Here's how the part is built. I have some questions about the finished solid (model axes, mm). A direction names the side the tool comes from. Coordinates: 2 decimals unless noted, no trailing zeros. Loops run counter-clockwise (first coordinate to the right, second up) from the corner with the lowest first, then second, coordinate; pieces in that order, holes last. Notation, with made-up numbers: (44, -27) - (70, -27) arc R24 ccw to (70, 7) - close; hole circle Ø6 at (43.5, 24). An arc over 180 degrees is marked (long way). Use a Markdown table: item, result.
```python
from build123d import *

# Parameters (mm, degrees)
F0_W     = 90
F0_H     = 90
F1_DEPTH = 3
F0_H_2   = 30
F2_DEPTH = 90
F3_DEPTH = 100
F4_DEPTH = 80


with BuildPart() as f1:
    # F0 (on Right) → F1 (new body)
    with BuildSketch(Plane.YZ):
        Polygon((264.885695, 154.677426), (34.885695, 154.677426), (34.885695, 0.538323), (199.884153, 0.538323), (199.884153, -1.461677), (163.329955, -1.461677), (163.329955, -31.461677), (73.329955, -31.461677), (73.329955, -1.461677), (34.885695, -1.461677), (34.885695, -75.322574), (264.885695, -75.322574), align=None)
        with Locations((96.11488, 95.538323)):
            Rectangle(F0_W, F0_H, mode=Mode.SUBTRACT)
    extrude(amount=F1_DEPTH)

    # F0 (on Right) → F2 (join)
    with BuildSketch(Plane.YZ):
        with Locations((118.329955, -16.461677)):
            Rectangle(F0_W, F0_H_2)
    extrude(amount=F2_DEPTH)

    # F0 (on Right) → F3 (join)
    with BuildSketch(Plane.YZ):
        Polygon((199.884153, 0.538323), (34.885695, 0.538323), (34.885695, -1.461677), (73.329955, -1.461677), (163.329955, -1.461677), (199.884153, -1.461677), align=None)
    extrude(amount=F3_DEPTH)

    # F0 (on Right) → F4 (join)
    with BuildSketch(Plane.YZ):
        with Locations((96.11488, 95.538323)):
            Rectangle(F0_W, F0_H)
    extrude(amount=F4_DEPTH)


solid = f1.part
```
Q1. I want a section at D-D, the plane z = 105.5. Write out the boundary of the cut face in (x, y), then the cut area to 3 significant figures.
Check values:
| item | result |
|---|---|
| outline | (0, 34.89) - (3, 34.89) - (3, 51.11) - (80, 51.11) - (80, 141.11) - (3, 141.11) - (3, 264.89) - (0, 264.89) - close |
| area | 7,620 mm^2 |
Q2. Will these pins go through, and if not, where does the flat tip stop? P1, Ø1, axis at x = 43.5, z = -1, coming from the +Y side; P2, Ø24, axis at x = 55, z = -16, coming from the +Y side; P3, Ø12, axis at x = 39.5, y = 165.5, coming from the +Z side.
Check values:
| item | result |
|---|---|
| P1 | y = 199.88 |
| P2 | y = 163.33 |
| P3 | z = 0.54 |
Q3. Which directions (+Z, -Z, +X, -X, +Y, -Y) give clear straight access to the entire face, cutting with the end or side of a thin tool? Please do faces 5 (the face through (46, 73.33, -17)), 6 (the face through (80, 95, 96)), 7 (the face through (41, 51.115, 95)), 8 (the face through (46, 163.33, -17)), 9 (the face through (46, 118, -31.462)).
Check values:
| item | result |
|---|---|
| face 5 | -Z, +X, -Y |
| face 6 | +Z, +X, +Y, -Y |
| face 7 | +Z, +X, -Y |
| face 8 | -Z, +X, +Y |
| face 9 | -Z, +X, +Y, -Y |
Q4. I want a section at B-B, the plane z = -23.5. Write out the boundary of the cut face in (x, y), then the cut area to 3 significant figures.
Check values:
| item | result |
|---|---|
| outline | (0, 34.89) - (3, 34.89) - (3, 73.33) - (90, 73.33) - (90, 163.33) - (3, 163.33) - (3, 264.89) - (0, 264.89) - close |
| area | 8,520 mm^2 |
Q5. If we mould it in two halves opening along Z, with no side actions, what happens to faces 1 (the face through (51, 119, 0.538)), 2 (the face through (0, 148, 41)), 3 (the face through (41, 95, 50.538)), 4 (the face through (41, 95, 140.538))? For each: pulls with the +Z half, pulls with the -Z half, needs draft (parallel to the pull), parting line crosses it, or undercut.
Check values:
| item | result |
|---|---|
| face 1 | undercut |
| face 2 | needs draft |
| face 3 | undercut |
| face 4 | pulls with the +Z half |
Q6. Please list where these lines run through material, in increasing order: L1, parallel to Z at x = 25, y = 127; L2, parallel to X at y = 81, z = 13; L3, parallel to Y at x = 62.5, z = 83. Write a range as from..to.
Check values:
| item | result |
|---|---|
| L1 | -31.46..0.54, 50.54..140.54 |
| L2 | 0..3 |
| L3 | 51.11..141.11 |
Q7. I want a section at C-C, the plane y = 106.5. Write out the boundary of the cut face in (x, z).
Check values:
| item | result |
|---|---|
| outline | (0, -75.32) - (3, -75.32) - (3, -31.46) - (90, -31.46) - (90, -1.46) - (100, -1.46) - (100, 0.54) - (3, 0.54) - (3, 50.54) - (80, 50.54) - (80, 140.54) - (3, 140.54) - (3, 154.68) - (0, 154.68) - close |
Q8. I want a section at A-A, the plane x = 46.5. Write out the boundary of the cut face in (y, z), then the cut area to 3 significant figures.
Check values:
| item | result |
|---|---|
| outline | (34.89, -1.46) - (73.33, -1.46) - (73.33, -31.46) - (163.33, -31.46) - (163.33, -1.46) - (199.88, -1.46) - (199.88, 0.54) - (34.89, 0.54) - close; (51.11, 50.54) - (141.11, 50.54) - (141.11, 140.54) - (51.11, 140.54) - close |
| area | 11,100 mm^2 |
